```python
from build123d import *

# Parameters (mm, degrees)
F0_R     = 15
F1_DEPTH = 50
F2_DEPTH = 15


with BuildPart() as f1:
    # F0 (on Front) → F1 (new body)
    with BuildSketch(Plane.XZ):
        with BuildLine():
            ThreePointArc((0, -30), (21.2132034356, -21.2132034356), (30, 0))
            ThreePointArc((30, 0), (21.2132034356, 21.2132034356), (0, 30))
            Line((0, 30), (-9.6060024019, 28.4204981986))
            ThreePointArc((-9.6060024019, 28.4204981986), (-30, 0), (-9.6060024019, -28.4204981986))
            Line((-9.6060024019, -28.4204981986), (0, -30))
        make_face()
        Circle(F0_R, mode=Mode.SUBTRACT)
    extrude(amount=F1_DEPTH)

    # F0 (on Front) → F2 (join)
    with BuildSketch(Plane.XZ):
        with BuildLine():
            ThreePointArc((-9.6060024019, -28.4204981986), (-30, 0), (-9.6060024019, 28.4204981986))
            Line((-9.6060024019, 28.4204981986), (-92.4337484988, 14.8012454964))
            ThreePointArc((-92.4337484988, 14.8012454964), (-80.2919164477, 11.4347327796), (-75, 0))
            ThreePointArc((-75, 0), (-80.2919164477, -11.4347327796), (-92.4337484988, -14.8012454964))
            Line((-92.4337484988, -14.8012454964), (-9.6060024019, -28.4204981986))
        make_face()
        with BuildLine():
            ThreePointArc((-75, 0), (-80.2919164477, 11.4347327796), (-92.4337484988, 14.8012454964))
            ThreePointArc((-92.4337484988, 14.8012454964), (-105, 0), (-92.4337484988, -14.8012454964))
            ThreePointArc((-92.4337484988, -14.8012454964), (-80.2919164477, -11.4347327796), (-75, 0))
        make_face()
    extrude(amount=F2_DEPTH)


solid = f1.part
```
Work out the finished part from the listing and answer in its coordinate system (mm). Coordinates: 2 decimals unless noted, no trailing zeros. Write each loop counter-clockwise with the first axis right and the second up, starting at its lowest first coordinate (ties: lowest second). Pieces come first, ordered by that corner, then holes.
Q1. A cutting plane is placed at B-B, the plane z = 0. Give the vertices of the cut face in (x, y).
Q2. Find the intervals of material crossed by line 1 (Y direction, x = -36, z = -9.5); line 2 (Z direction, x = -5, y = -19.5); line 3 (X direction, y = -34, z = -11.5), in increasing order.
Q3. A cutting plane is placed at A-A, the plane y = -22. Give the vertices of the cut face in (x, z), then the cut area to 3 significant figures.
Q4. A cutting plane is placed at D-D, the plane x = -91. Give the vertices of the cut face in (y, z).
Q5. Determine the mould class of faces 1 (the face through (-29.995, -32.255, 0.523)), 2 (the face through (-14.985, -24.65, 0.66)), 3 (the face through (-58, -15, 0)) for opening direction X: released by +X, released by -X, zero draft, split by the parting line, or undercut.
Q6. A cutting plane is placed at C-C, the plane z = -24. Give the vertices of the cut face in (x, y).
Q7. Each of these flat-tipped pins is pushed along its axis until it touches: pin 1 Ø6 at (y, z) = (-35, 5) entering from +X; pin 2 Ø6 at (x, y) = (-82.5, -9.5) entering from -Z; pin 3 Ø10 at (x, y) = (-27, -7.5) entering from -Z. Where does it stop, or does it pass through?
Findings below:
1. outline: (-105, -15) - (-30, -15) - (-30, -50) - (-15, -50) - (-15, 0) - (-105, 0) - close; (15, -50) - (30, -50) - (30, 0) - (15, 0) - close
2. line 1: y = -15 to 0
2. line 2: z = -29.18 to -14.14, 14.14 to 29.18
2. line 3: x = -27.71 to -9.63, 9.63 to 27.71
3. outline: (-9.61, -28.42) - (0, -30) arc R30 ccw to (0, 30) - (-9.61, 28.42) arc R30 ccw to start; hole circle Ø30 at (0, 0)
3. area: 2,120 mm2
4. outline: (-15, -15.04) - (0, -15.04) - (0, 15.04) - (-15, 15.04) - close
5. face 1: released by -X
5. face 2: undercut
5. face 3: zero draft
6. outline: (-36.49, -15) - (-18, -15) - (-18, -50) - (18, -50) - (18, 0) - (-36.49, 0) - close
7. pin 1: stops at x = 29.93
7. pin 2: stops at z = -16.93
7. pin 3: stops at z = -26.38
